Source: CAD feature listing. Evaluate the final solid. Frame: model axes, mm. A direction names the side the tool comes from. Give positions to 0.01 mm unless a question says otherwise; leave off trailing zeros. Loops run counter-clockwise (first coordinate to the right, second up) from the corner with the lowest first, then second, coordinate; pieces in that order, holes last. Notation, with made-up numbers: (-17, 81) -> (-2, 81) arc R9 ccw to (-2, 86) -> close; hole circle Ø5 at (-37, -11.75). An arc over 180 degrees is marked (long way). Put each result on its own line as item: value.
```python
from build123d import *

# Parameters (mm, degrees)
SKETCH1_W                                      = 57.15
SKETCH1_H                                      = 43.18
BASE_DEPTH                                     = 57.15
SKETCH2_W                                      = 52.07
SKETCH2_H                                      = 38.1
POCKET_DEPTH                                   = 47.9552
SKETCH3_W                                      = 18.288
SKETCH3_H                                      = 15.494
LINACTHOLE_DEPTH                               = 68.44465305
ROLLMOTORHOLE_REACH                            = 85.656
SKETCH4_W                                      = 20.066
SKETCH4_H                                      = 9.525
DVIHOLE_REACH                                  = 69.445
CBORE_FOR_4_SOCKET_HEAD_CAP_SCREW1_D           = 3.2639
CBORE_FOR_4_SOCKET_HEAD_CAP_SCREW1_CBORE_D     = 5.55752
CBORE_FOR_4_SOCKET_HEAD_CAP_SCREW1_CBORE_DEPTH = 2.8448
CBORE_FOR_8_SOCKET_HEAD_CAP_SCREW1_D           = 4.4958
CBORE_FOR_8_SOCKET_HEAD_CAP_SCREW1_CBORE_D     = 7.9375
CBORE_FOR_8_SOCKET_HEAD_CAP_SCREW1_CBORE_DEPTH = 4.1656
FILLET1_R                                      = 0.254


with BuildPart() as part:
    # Sketch1 → Base (new body)
    with BuildSketch(Plane(origin=(0, 0, 0), x_dir=(1, 0, 0), z_dir=(0, 1, 0))):
        Rectangle(SKETCH1_W, SKETCH1_H)
    extrude(amount=BASE_DEPTH)

    # Sketch2 → Pocket (cut)
    with BuildSketch(Plane(origin=(0, 57.15, 0), x_dir=(1, 0, 0), z_dir=(0, 1, 0))):
        Rectangle(SKETCH2_W, SKETCH2_H)
    extrude(amount=-POCKET_DEPTH, mode=Mode.SUBTRACT)

    # Sketch3 → LinActHole (cut, through all)
    with BuildSketch(Plane(origin=(0, 0, 0), x_dir=(-1, 0, 0), z_dir=(0, -1, 0))):
        with Locations((-1.651, 0)):
            Rectangle(SKETCH3_W, SKETCH3_H)
    extrude(amount=-LINACTHOLE_DEPTH, mode=Mode.SUBTRACT)

    # Sketch4 → RollMotorHole (cut, up to next)
    with BuildSketch(Plane.ZY.offset(28.575), mode=Mode.PRIVATE) as rollmotorhole_sk1:
        with Locations((5.715, 52.3875)):
            Rectangle(SKETCH4_W, SKETCH4_H)
    rollmotorhole_tool1 = extrude(rollmotorhole_sk1.sketch, amount=-ROLLMOTORHOLE_REACH, mode=Mode.PRIVATE) & part.part
    add(rollmotorhole_tool1.solids().sort_by_distance((-28.575, 52.3875, 5.715))[0], mode=Mode.SUBTRACT)

    # Sketch5 → DviHole (cut, up to next)
    with BuildSketch(Plane.XZ, mode=Mode.PRIVATE) as dvihole_sk1:
        with BuildLine():
            Line((17.624947543, -13.716), (24.228947543, -13.716))
            Line((24.228947543, -13.716), (24.228947543, 13.716))
            Line((24.228947543, 13.716), (17.624947543, 13.716))
            ThreePointArc((17.624947543, 13.716), (15.828896319, 12.972051224), (15.084947543, 11.176))
            Line((15.084947543, 11.176), (15.084947543, -11.176))
            ThreePointArc((15.084947543, -11.176), (15.828896319, -12.972051224), (17.624947543, -13.716))
        make_face()
    dvihole_tool1 = extrude(dvihole_sk1.sketch, amount=-DVIHOLE_REACH, mode=Mode.PRIVATE) & part.part
    add(dvihole_tool1.solids().sort_by_distance((19.701649, 0, 0))[0], mode=Mode.SUBTRACT)

    # CBORE for #4 Socket Head Cap Screw1 (through all)
    with Locations(Plane(origin=(0, 0, 0), x_dir=(-1, 0, 0), z_dir=(0, -1, 0))):
        with Locations((-19.656947543, 16.256), (-19.656947543, -16.256)):
            CounterBoreHole(CBORE_FOR_4_SOCKET_HEAD_CAP_SCREW1_D / 2, CBORE_FOR_4_SOCKET_HEAD_CAP_SCREW1_CBORE_D / 2, CBORE_FOR_4_SOCKET_HEAD_CAP_SCREW1_CBORE_DEPTH)

    # CBORE for #8 Socket Head Cap Screw1 (through all)
    with Locations(Plane(origin=(0, 0, 0), x_dir=(-1, 0, 0), z_dir=(0, -1, 0))):
        with Locations((3.175, 14.605), (3.175, -14.605)):
            CounterBoreHole(CBORE_FOR_8_SOCKET_HEAD_CAP_SCREW1_D / 2, CBORE_FOR_8_SOCKET_HEAD_CAP_SCREW1_CBORE_D / 2, CBORE_FOR_8_SOCKET_HEAD_CAP_SCREW1_CBORE_DEPTH)

    # Fillet1
    fillet1_edges = [part.edges().sort_by_distance(p)[0] for p in [
        (20.783849108, 1.4224, 13.716),
        (18.530045978, 1.4224, 13.716),
        (18.530045978, 1.4224, -13.716),
        (20.783849108, 1.4224, -13.716),
    ]]
    fillet(fillet1_edges, radius=FILLET1_R)


solid = part.part
```
(1) Section D-D on y = 7. Return loops of the section in (x, z) (3 decimals), then the cut area to 3 significant figures.
Calculated:
outline: (-28.575, -21.59) -> (28.575, -21.59) -> (28.575, 21.59) -> (-28.575, 21.59) -> close; hole (-7.493, -7.747) -> (10.795, -7.747) -> (10.795, 7.747) -> (-7.493, 7.747) -> close; hole circle Ø4.496 at (-3.175, -14.605); hole circle Ø4.496 at (-3.175, 14.605); hole (15.085, -11.176) arc R2.54 ccw to (17.625, -13.716) -> (24.229, -13.716) -> (24.229, 13.716) -> (17.625, 13.716) arc R2.54 ccw to (15.085, 11.176) -> close; hole circle Ø3.264 at (19.657, -16.256); hole circle Ø3.264 at (19.657, 16.256)
area: 1,890 mm²
(2) First-contact query: P1, Ø4, axis at x = 19.66, z = -16.26, coming from the -Y side; P2, Ø7, axis at x = -3.175, z = -14.605, coming from the +Y side; P3, Ø7, axis at x = -3.175, z = 14.605, coming from the -Y side. Flat tips, straight axial feed; report the tip coordinate or a pass-through.
Calculated:
P1: stops at y = 2.84
P2: stops at y = 9.19
P3: stops at y = 4.17
(3) Line query: probe 1 along X at (y, z) = (40, 9) (3 decimals); probe 2 along Z at (x, y) = (-13, 24); probe 3 along X at (y, z) = (3.5, 11.5) (3 decimals). Output: solid intervals per line, ascending. Write a range as from..to.
Calculated:
probe 1: x = -28.575..-26.035, 26.035..28.575
probe 2: z = -21.59..-19.05, 19.05..21.59
probe 3: x = -28.575..-5.647, -0.703..15.106, 24.229..28.575
(4) Section B-B on y = 46.5. Return loops of the section in (x, z) (3 decimals), then the cut area to 3 significant figures.
Calculated:
outline: (-28.575, -21.59) -> (28.575, -21.59) -> (28.575, 21.59) -> (-28.575, 21.59) -> close; hole (-26.035, -19.05) -> (26.035, -19.05) -> (26.035, 19.05) -> (-26.035, 19.05) -> close
area: 484 mm²
(5) Reachability of faces 4 (the flat face through (26.035, 34, 0)), 5 (the cylindrical face through (19.563, 1.402, -19.033)), 6 (the flat face through (-27, 52, 15.748)), 7 (the flat face through (2, 5, -7.747)) from +Z, -Z, +X, -X, +Y, -Y: full face, straight path, thin tool, end or side. Return the list, or none.
Calculated:
face 4: +Y
face 5: -Y
face 6: -X, +Y
face 7: +Y, -Y
(6) Section A-A on z = -7. Return loops of the section in (x, y) (3 decimals), then the cut area to 3 significant figures.
Calculated:
outline: (-28.575, 0) -> (-7.493, 0) -> (-7.493, 9.195) -> (-26.035, 9.195) -> (-26.035, 57.15) -> (-28.575, 57.15) -> close; (10.795, 0) -> (15.085, 0) -> (15.085, 9.195) -> (10.795, 9.195) -> close; (24.229, 0) -> (28.575, 0) -> (28.575, 57.15) -> (26.035, 57.15) -> (26.035, 9.195) -> (24.229, 9.195) -> close
area: 517 mm²
(7) Draft query along X for faces 1 (the flat face through (28.575, 28, 0)), 2 (the flat face through (10.795, 5, 0)), 3 (the flat face through (-27, 47.625, 6)). Return one class per face: released by +X, released by -X, zero draft, split by the parting line, or undercut.
Calculated:
face 1: released by +X
face 2: undercut
face 3: zero draft
(8) Section C-C on x = -2.5. Return loops of the section in (y, z), then the cut area to 3 significant figures.
Calculated:
outline: (0, -21.59) -> (57.15, -21.59) -> (57.15, -19.05) -> (9.19, -19.05) -> (9.19, -16.75) -> (4.17, -16.75) -> (4.17, -18.52) -> (0, -18.52) -> close; (0, -10.69) -> (4.17, -10.69) -> (4.17, -12.46) -> (9.19, -12.46) -> (9.19, -7.75) -> (0, -7.75) -> close; (0, 7.75) -> (9.19, 7.75) -> (9.19, 12.46) -> (4.17, 12.46) -> (4.17, 10.69) -> (0, 10.69) -> close; (0, 18.52) -> (4.17, 18.52) -> (4.17, 16.75) -> (9.19, 16.75) -> (9.19, 19.05) -> (57.15, 19.05) -> (57.15, 21.59) -> (0, 21.59) -> close
area: 390 mm²
